Autodesk Inventor part; units mm, degrees
ref_plane "YZ Plane" through (0, 0, 0) normal (1, 0, 0) x (0, 1, 0)
ref_plane "XZ Plane" through (0, 0, 0) normal (0, 1, 0) x (-1, 0, 0)
ref_plane "XY Plane" through (0, 0, 0) normal (0, 0, 1) x (1, 0, 0)
sketch "Esquisse1" plane through (0, 0, 0) normal (0, 0, 1) x (1, 0, 0)
  line L0 (-65.5174, -57.3571) -> (-65.5174, -54.3571) construction
  line L1 (-65.5174, -57.3571) -> (68.5174, -57.3571) construction
  line L2 (68.5174, -54.3571) -> (68.5174, -57.3571) construction
  line L3 (68.5174, -54.3571) -> (-65.5174, -54.3571) construction
  line L4 (-65.5174, -65.3571) -> (-65.5174, -62.3571) construction
  line L5 (-65.5174, -65.3571) -> (68.5174, -65.3571) construction
  line L6 (68.5174, -62.3571) -> (68.5174, -65.3571) construction
  line L7 (68.5174, -62.3571) -> (-65.5174, -62.3571) construction
  line L8 (68.5174, -54.3571) -> (-65.5174, -65.3571) construction
  line L9 (-65.5174, -54.3571) -> (68.5174, -65.3571) construction
  line L10 (-65.5174, -61.8571) -> (68.5174, -61.8571)
  line L11 (68.5174, -61.8571) -> (68.5174, -57.8571)
  line L12 (68.5174, -57.8571) -> (-65.5174, -57.8571)
  line L13 (-65.5174, -57.8571) -> (-65.5174, -61.8571)
  line L14 (-65.5174, -61.8571) -> (68.5174, -57.8571) construction
  line L15 (68.5174, -61.8571) -> (-65.5174, -57.8571) construction
  line L16 (68.5174, -54.3571) -> (18.5174, -54.3571)
  line L17 (18.5174, -54.3571) -> (18.5174, -51.3571)
  line L18 (18.5174, -51.3571) -> (68.5174, -51.3571)
  line L19 (68.5174, -51.3571) -> (68.5174, -54.3571)
  line L20 (68.5174, -65.3571) -> (18.5174, -65.3571)
  line L21 (18.5174, -65.3571) -> (18.5174, -68.3571)
  line L22 (18.5174, -68.3571) -> (68.5174, -68.3571)
  line L23 (68.5174, -68.3571) -> (68.5174, -65.3571)
  line L24 (18.5174, -57.8571) -> (18.5174, -61.8571)
  point P0 (0, 0)
  point P1 (1.5, -59.8571)
  dimension "d1" = 0.5
  dimension "d2" = 50
  dimension "d3" = 3
  dimension "d4" = 3
extrude "Extrusion1" add sketch "Esquisse1" along normal blind 2.9 contours L24 L12 L11 L10 | L16 L17 L18 L19 | L23 L22 L21 L20
sketch "Esquisse13" plane through (0, 0, 0) normal (0, 0, -1) x (-1, 0, 0)
  line L0 (-68.5174, -68.3571) -> (-68.5174, -65.3571)
  line L1 (-18.5174, -51.3571) -> (-68.5174, -51.3571)
  line L2 (-68.5174, -51.3571) -> (-68.5174, -68.3571)
  line L3 (-68.5174, -68.3571) -> (-18.5174, -68.3571)
  line L4 (-18.5174, -68.3571) -> (-18.5174, -51.3571)
  point P0 (0, 0)
extrude "Extrusion12" add sketch "Esquisse13" along normal blind 2
sketch "Esquisse24" plane through (0, 0, -2) normal (0, 0, -1) x (-1, 0, 0)
  line L0 (-18.5174, -65.3571) -> (-18.5174, -68.3571)
  line L1 (-18.5174, -51.3571) -> (-68.5174, -51.3571)
  line L2 (-18.5174, -68.3571) -> (-68.5174, -68.3571)
  line L3 (-68.5174, -68.3571) -> (-68.5174, -51.3571)
  line L4 (-68.5174, -51.3571) -> (-18.5174, -51.3571)
  line L5 (-18.5174, -51.3571) -> (-18.5174, -68.3571)
  point P0 (0, 0)
extrude "Extrusion21" add sketch "Esquisse24" along normal blind 5
sketch "Esquisse25" plane through (18.5174, -68.3571, 2.9) normal (0, -1, 0) x (1, 0, 0)
  line L0 (50, -9.9) -> (50, 0)
  line L1 (50, -9.9) -> (0, -9.9)
  line L2 (0, -9.9) -> (0, -4.95)
  line L3 (0, -4.95) -> (50, -4.95)
  line L4 (50, -4.95) -> (50, -9.9)
  line L5 (0, -9.9) -> (0, 0) construction
  point P0 (-18.5174, -2.9)
extrude "Extrusion22" add sketch "Esquisse25" along normal blind 15
sketch "Esquisse26" plane through (18.5174, -68.3571, -2.05) normal (0, 0, 1) x (1, 0, 0)
  line L0 (50, -15) -> (0, -15)
  line L1 (0, 0) -> (50, 0)
  line L2 (0, -15) -> (50, 0)
  line L3 (0, 0) -> (50, -15)
  line L4 (25, -7.5) -> (25, -60)
  circle A0 centre (25, -60) radius 45
  line L5 (0, -15) -> (50, -15)
  line L6 (0, -15) -> (0, -22.5834)
  line L7 (50, 0) -> (50, -15)
  line L8 (50, -15) -> (50, -22.5834)
  line L9 (0, -15) -> (25, -15)
  line L10 (25, -15) -> (50, -15)
  point P0 (-18.5174, 68.3571)
  dimension "d89" = 90
extrude "Extrusion23" add sketch "Esquisse26" against normal up to surface (4.95 mm away) contours L8 A0 L0 | A0 L6 L0 | A0
sketch "Esquisse27" plane through (0, 0, -7) normal (0, 0, -1) x (-1, 0, 0)
  line L0 (-18.5174, -51.3571) -> (-18.5174, -90.9406)
  line L1 (-18.5174, -51.3571) -> (-68.5174, -51.3571)
  line L2 (-68.5174, -51.3571) -> (-68.5174, -90.9406)
  arc A0 (-68.5174, -90.9406) -> (-18.5174, -90.9406) centre (-43.5174, -128.3571) ccw
  point P0 (0, 0)
extrude "Extrusion24" cut sketch "Esquisse27" against normal blind 2.5
sketch "Esquisse28" plane through (18.5174, -68.3571, -2.05) normal (0, 0, 1) x (1, 0, 0)
  arc A0 (0, -22.5834) -> (50, -22.5834) centre (25, -60) ccw construction
  line L0 (25, -60) -> (-20, -60)
  point P0 (-18.5174, 68.3571)
ref_plane "Plan de construction5" through (43.5174, -128.3571, -2.05) normal (0, -1, 0) x (1, 0, 0)
ref_plane "Plan de construction6" through (43.5174, -128.3571, -2.05) normal (-1, 0, 0) x (0, -1, 0)
sketch "Esquisse29" plane through (0, 0, -4.5) normal (0, 0, -1) x (-1, 0, 0)
  circle A0 centre (-29.1178, -158.4374) radius 1.5
  circle A1 centre (-24.1083, -100.8982) radius 1.5
  circle A2 centre (-76.4793, -125.6998) radius 1.5
  point P0 (0, 0)
extrude "Extrusion25" cut sketch "Esquisse29" against normal blind 15
sketch "Esquisse30" plane through (18.5174, -68.3571, -2.05) normal (0, 0, 1) x (1, 0, 0)
  circle A0 centre (57.9619, -57.3427) radius 1.5
  circle A1 centre (10.6003, -90.0802) radius 1.5
  circle A2 centre (5.5909, -32.541) radius 1.5
  line L0 (0, 0) -> (50, 0)
  line L1 (0, 0) -> (0, -22.5834)
  arc A3 (0, -22.5834) -> (50, -22.5834) centre (25, -60) ccw
  line L2 (50, 0) -> (50, -22.5834)
  line L3 (50, -22.5834) -> (50, 17)
  line L4 (50, -22.5834) -> (0, -22.5834)
  point P0 (-18.5174, 68.3571)
  point P1 (0, -22.5834)
extrude "Extrusion26" add sketch "Esquisse30" along normal blind 10 contours L4 A3
sketch "Esquisse31" plane through (0, 0, -4.5) normal (0, 0, -1) x (-1, 0, 0)
  line L0 (-97.6483, -128.3571) -> (22.3325, -128.3571)
  line L1 (-43.5174, -178.8817) -> (-43.5174, -79.6766)
  circle A0 centre (-43.5174, -128.3571) radius 43
  arc A1 (-68.5174, -90.9406) -> (-18.5174, -90.9406) centre (-43.5174, -128.3571) ccw
  line L2 (-68.5174, -68.3571) -> (-68.5174, -90.9406)
  line L3 (-68.5174, -90.9406) -> (-18.5174, -90.9406)
  point P0 (0, 0)
  point P1 (-64.707, -90.9406)
  point P2 (-22.3278, -90.9406)
  dimension "d98" = 2
sketch "Esquisse34" plane through (18.5174, -68.3571, 7.95) normal (0, 0, 1) x (1, 0, 0)
  arc A0 (0, -22.5834) -> (50, -22.5834) centre (25, -60) ccw
  line L0 (50, -22.5834) -> (0, -22.5834)
  circle A1 centre (5.5909, -32.541) radius 1.5
  circle A2 centre (10.6003, -90.0802) radius 1.5
  circle A3 centre (57.9619, -57.3427) radius 1.5
  arc A4 (0.6142, -24.5834) -> (49.3858, -24.5834) centre (25, -60) ccw
  line L1 (0.6142, -24.5834) -> (49.3858, -24.5834)
  point P0 (-18.5174, 68.3571)
  dimension "d103" = 2
extrude "Extrusion29" cut sketch "Esquisse34" against normal blind 10 contours L1 A4
sketch "Esquisse35" plane through (43.5174, -128.3571, -2.05) normal (-1, 0, 0) x (0, -1, 0)
  line L0 (0, 9.1389) -> (0, 21.1265) construction
  circle A0 centre (0, 15.1327) radius 2
  point P0 (-128.3571, 2.05)
  dimension "d106" = 4
properties part number "rainHolder_Impression 3D"
Part model, mm, in its own coordinate system. A direction names the side the tool comes from. Give positions to 0.01 mm unless a question says otherwise; leave off trailing zeros. Order: outer loops, then holes, each group sorted by start corner. A loop starts at its lowest first (then second) coordinate and runs counter-clockwise, first axis right, second up. Notation, with made-up numbers: M 72,86 L 82,86 A18 cw 82,105 Z; hole C 54,67 d6. An arc over 180 degrees is marked long. Use a Markdown table: item, result. Add a question column.
(1) 3-axis set-ups, long thin cutter, end or side, ignore diameter. For faces 1 (the face through (43, -79, -2.05)), 2 (the face through (43, -132, -2.05)), 3 (the face through (68.517, -66, -2)): which of +Z, -Z, +X, -X, +Y, -Y reach the whole face in a straight line?
(2) Saw through at B-B, the plane z = 6.5. Give the cut face in (x, y).
(3) Saw through at D-D, the plane x = 39.5. Give the cut face in (y, z), and give its area (3 significant figures).
(4) Saw through at C-C, the plane y = -132. Give the cut face in (x, z), and give its area (3 significant figures).
(5) Drop flat-ended pins along their axis: P1, Ø3, axis at x = 51, z = 2, coming from the -Y side; P2, Ø3.5, axis at x = 40, y = -53.5, coming from the +Z side; P3, Ø1, axis at x = 47.5, y = -56, coming from the +Z side. Give the stop position or say it passes through.
(6) Probe line 1 along Y through (x, z) = (65, -1); line 2 along Y through (x, z) = (53, -1); line 3 along Y through (x, z) = (56, 2). List the from-to ranges inside material, lowest first. Write a range as [from, to].
(7) Mould opens along X. For faces 4 (the face through (41.99, -171.33, 3.02)), 5 (the face through (43, -92, 7.95)), 6 (the face through (45.13, -173.33, 2.88)) say: +X half, -X half, draft (parallel to the pull), parting line (faces both ways), or undercut.
(8) Saw through at A-A, the plane x = 51.5. Give the cut face in (y, z), and give its area (3 significant figures).
Answer key:
| question | item | result |
|---|---|---|
| 1 | face 1 | +Z, +X, -X |
| 1 | face 2 | +Z |
| 1 | face 3 | +Z, -Z, +X, +Y |
| 2 | outline | M 18.52,-90.94 A45 ccw long 68.52,-90.94 Z; hole M 19.13,-92.94 A43 ccw long 67.9,-92.94 Z |
| 3 | outline | M -173.18,-4.5 L -51.36,-4.5 L -51.36,2.9 L -54.36,2.9 L -54.36,0 L -57.86,0 L -57.86,2.9 L -61.86,2.9 L -61.86,0 L -65.36,0 L -65.36,2.9 L -68.36,2.9 L -68.36,-2.05 L -90.94,-2.05 L -90.94,7.95 L -92.94,7.95 L -92.94,-2.05 L -171.17,-2.05 L -171.17,7.95 L -173.18,7.95 Z |
| 3 | area | 402 mm^2 |
| 4 | outline | M -1.33,-4.5 L 88.37,-4.5 L 88.37,7.95 L 86.36,7.95 L 86.36,-2.05 L 0.67,-2.05 L 0.67,7.95 L -1.33,7.95 Z |
| 4 | area | 260 mm^2 |
| 5 | P1 | y = -172.96 |
| 5 | P2 | z = 2.9 |
| 5 | P3 | z = 0 |
| 6 | line 1 | [-167.9, -165.61], [-92.94, -90.94], [-68.36, -51.36] |
| 6 | line 2 | [-172.35, -170.3], [-92.94, -90.94], [-68.36, -51.36] |
| 6 | line 3 | [-171.59, -169.51], [-92.94, -90.94], [-68.36, -65.36], [-61.86, -57.86], [-54.36, -51.36] |
| 7 | face 4 | undercut |
| 7 | face 5 | draft |
| 7 | face 6 | parting line |
| 8 | outline | M -172.64,-4.5 L -51.36,-4.5 L -51.36,2.9 L -54.36,2.9 L -54.36,0 L -57.86,0 L -57.86,2.9 L -61.86,2.9 L -61.86,0 L -65.36,0 L -65.36,2.9 L -68.36,2.9 L -68.36,-2.05 L -90.94,-2.05 L -90.94,7.95 L -92.94,7.95 L -92.94,-2.05 L -170.61,-2.05 L -170.61,7.95 L -172.64,7.95 Z |
| 8 | area | 401 mm^2 |
